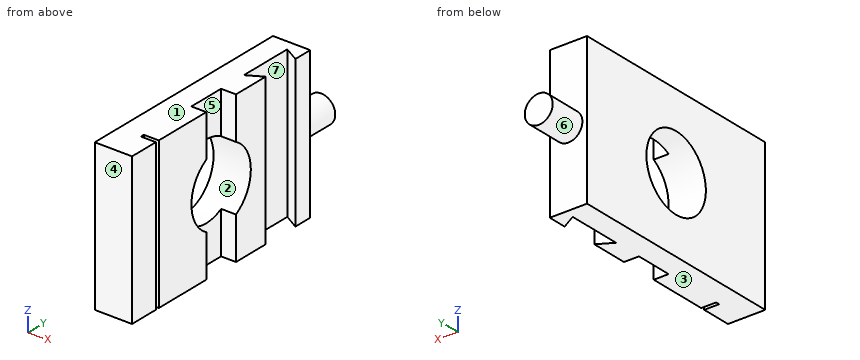
```python
from build123d import *

# Parameters (mm, degrees)
F0_W     = 76.2
F0_H     = 50.8
F0_R     = 12.7
F1_DEPTH = 12.7
F2_W     = 1.27
F2_H     = 50.8
F3_DEPTH = 5.08
F5_DEPTH = 50.801
F6_R     = 4.7625
F7_DEPTH = 12.7


with BuildPart() as f1:
    # F0 (on Right) → F1 (new body)
    with BuildSketch(Plane.YZ):
        with Locations((36.5860867262, -18.7051647067)):
            Rectangle(F0_W, F0_H)
        with Locations((36.5860867262, -18.7051647067)):
            Circle(F0_R, mode=Mode.SUBTRACT)
    extrude(amount=F1_DEPTH)

    # F2 (on face) → F3 (cut)
    with BuildSketch(Plane.YZ.offset(12.7)):
        with Locations((9.2810867262, -18.7051647067)):
            Rectangle(F2_W, F2_H)
        with BuildLine():
            Line((42.9360867262, 6.6948352933), (30.2360867262, 6.6948352933))
            Line((30.2360867262, 6.6948352933), (30.2360867262, -7.7066420786))
            ThreePointArc((30.2360867262, -7.7066420786), (36.5860867262, -6.0051647067), (42.9360867262, -7.7066420786))
            Line((42.9360867262, -7.7066420786), (42.9360867262, 6.6948352933))
        make_face()
        with BuildLine():
            Line((30.2360867262, -29.7036873348), (30.2360867262, -44.1051647067))
            Line((30.2360867262, -44.1051647067), (42.9360867262, -44.1051647067))
            Line((42.9360867262, -44.1051647067), (42.9360867262, -29.7036873348))
            ThreePointArc((42.9360867262, -29.7036873348), (36.5860867262, -31.4051647067), (30.2360867262, -29.7036873348))
        make_face()
    extrude(amount=-F3_DEPTH, mode=Mode.SUBTRACT)

    # F4 (on face) → F5 (cut, through all)
    with BuildSketch(Plane(origin=(0, 0, -44.1051647067), x_dir=(1, 0, 0), z_dir=(0, 0, -1))):
        Polygon((12.7, -68.3360867262), (12.7, -55.6360867262), (7.62, -52.7031473587), (7.62, -71.2690260937), align=None)
    extrude(amount=-F5_DEPTH, mode=Mode.SUBTRACT)

    # F6 (on face) → F7 (join)
    with BuildSketch(Plane(origin=(0, 74.6860867262, 0), x_dir=(-1, 0, 0), z_dir=(0, 1, 0))):
        with Locations((-6.35, -18.7051647067)):
            Circle(F6_R)
    extrude(amount=F7_DEPTH)


solid = f1.part
```
CAD build for the part. Positions are in the model's coordinates, mm. Face numbers are marked on the shaded views. A direction names the side the tool comes from. Round coordinates to 2 decimals unless told otherwise and drop trailing zeros. Write each loop counter-clockwise with the first axis right and the second up, starting at its lowest first coordinate (ties: lowest second). Pieces come first, ordered by that corner, then holes.
Item 1: Drop flat-ended pins along their axis: pin 1 Ø6 at (x, y) = (11.5, 38.5) entering from -Z (3 decimals); pin 2 Ø5 at (x, z) = (5, -26.5) entering from +Y; pin 3 Ø3 at (y, z) = (61, 0) entering from +X. Give the stop position or say it passes through.
Filled in:
pin 1: passes through
pin 2: stops at y = 74.69
pin 3: stops at x = 7.62
Item 2: Band-saw the part on B-B on y = 44. Write the cut outline in (x, z).
Filled in:
outline: (0, -44.11) - (12.7, -44.11) - (12.7, -29.02) - (0, -29.02) - close; (0, -8.39) - (12.7, -8.39) - (12.7, 6.69) - (0, 6.69) - close
Item 3: Band-saw the part on D-D on z = -39. Write the cut outline in (x, y), then the cut area to 3 significant figures.
Filled in:
outline: (0, -1.51) - (12.7, -1.51) - (12.7, 8.65) - (7.62, 8.65) - (7.62, 9.92) - (12.7, 9.92) - (12.7, 30.24) - (7.62, 30.24) - (7.62, 42.94) - (12.7, 42.94) - (12.7, 55.64) - (7.62, 52.7) - (7.62, 71.27) - (12.7, 68.34) - (12.7, 74.69) - (0, 74.69) - close
area: 817 mm2
Item 4: Mould opens along Z. For the marked faces 1, 2, 3 and 4 say: released by +Z, released by -Z, zero draft, split by the parting line, or undercut.
Filled in:
face 1: released by +Z
face 2: undercut
face 3: released by -Z
face 4: zero draft
Item 5: Drill centre lines: L1, parallel to Y at x = 9, z = -14; L2, parallel to Y at x = 10.25, z = -28; L3, parallel to Y at x = 1, z = -18. Where is each one in solid material? Low to high.
Filled in:
L1: y = -1.51 to 8.65, 9.92 to 24.79, 48.38 to 53.5, 70.47 to 74.69
L2: y = -1.51 to 8.65, 9.92 to 27.93, 45.24 to 54.22, 69.75 to 74.69
L3: y = -1.51 to 23.91, 49.27 to 74.69
Item 6: Band-saw the part on C-C on x = 6.35. Write the cut outline in (y, z).
Filled in:
outline: (-1.51, -44.11) - (74.69, -44.11) - (74.69, -23.47) - (87.39, -23.47) - (87.39, -13.94) - (74.69, -13.94) - (74.69, 6.69) - (-1.51, 6.69) - close; hole circle Ø25.4 at (36.59, -18.71)
Item 7: Band-saw the part on A-A on z = -22.5. Write the cut outline in (x, y), then the cut area to 3 significant figures.
Filled in:
outline: (0, -1.51) - (12.7, -1.51) - (12.7, 8.65) - (7.62, 8.65) - (7.62, 9.92) - (12.7, 9.92) - (12.7, 24.47) - (0, 24.47) - close; (0, 48.71) - (12.7, 48.71) - (12.7, 55.64) - (7.62, 52.7) - (7.62, 71.27) - (12.7, 68.34) - (12.7, 74.69) - (9.23, 74.69) - (9.23, 87.39) - (3.47, 87.39) - (3.47, 74.69) - (0, 74.69) - close
area: 647 mm2
Item 8: Tool access for the marked faces 5, 6 and 7: list every direction of +Z, -Z, +X, -X, +Y, -Y with a clear straight run to the whole face (end or side of a thin tool).
Filled in:
face 5: +Z, -Z, +X
face 6: +Y
face 7: +Z, -Z
